Part model, mm, in its own coordinate system. Give positions to 0.01 mm unless a question says otherwise; leave off trailing zeros. Write each loop counter-clockwise with the first axis right and the second up, starting at its lowest first coordinate (ties: lowest second). Pieces come first, ordered by that corner, then holes.
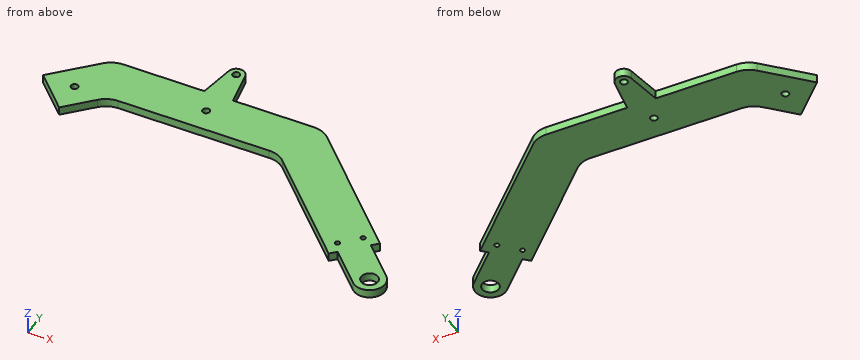
```python
from build123d import *

# Parameters (mm, degrees)
SKETCH5_R           = 1
SKETCH5_R_2         = 3.5
SKETCH5_R_3         = 1.5
BOSS_EXTRUDE1_DEPTH = 3.5
FILLET1_R           = 10


with BuildPart() as part:
    # Sketch5 → Boss-Extrude1 (new body)
    with BuildSketch(Plane.XY):
        with BuildLine():
            Line((91.161165235, 18.03122292), (104.596194078, 4.596194078))
            ThreePointArc((104.596194078, 4.596194078), (104.596194078, -4.596194078), (95.403805922, -4.596194078))
            Line((95.403805922, -4.596194078), (81.96877708, 8.838834765))
            Line((81.96877708, 8.838834765), (79.493903346, 6.363961031))
            Line((79.493903346, 6.363961031), (35.857864376, 50))
            Line((35.857864376, 50), (-35.857864376, 50))
            Line((-35.857864376, 50), (-49.445436483, 36.412427894))
            Line((-49.445436483, 36.412427894), (-63.587572106, 50.554563517))
            Line((-63.587572106, 50.554563517), (-44.142135624, 70))
            Line((-44.142135624, 70), (-6, 70))
            Line((-6, 70), (-3.448564481, 84.717831932))
            ThreePointArc((-3.448564481, 84.717831932), (0, 87.62), (3.448564481, 84.717831932))
            Line((3.448564481, 84.717831932), (6, 70))
            Line((6, 70), (44.142135624, 70))
            Line((44.142135624, 70), (93.636038969, 20.506096654))
            Line((93.636038969, 20.506096654), (91.161165235, 18.03122292))
        make_face()
        with Locations((86.564971157, 20.506096654)):
            Circle(SKETCH5_R, mode=Mode.SUBTRACT)
        with Locations((79.493903346, 13.435028843)):
            Circle(SKETCH5_R, mode=Mode.SUBTRACT)
        with Locations((100, 0)):
            Circle(SKETCH5_R_2, mode=Mode.SUBTRACT)
        with Locations((0, 84.12)):
            Circle(SKETCH5_R_3, mode=Mode.SUBTRACT)
        with Locations((0, 60)):
            Circle(SKETCH5_R_3, mode=Mode.SUBTRACT)
        with Locations((-50, 50)):
            Circle(SKETCH5_R_3, mode=Mode.SUBTRACT)
    extrude(amount=BOSS_EXTRUDE1_DEPTH)

    # Fillet1
    fillet1_edges = [part.edges().sort_by_distance(p)[0] for p in [
        (44.142135624, 70, 1.75),
        (35.857864376, 50, 1.75),
        (-35.857864376, 50, 1.75),
        (-44.142135624, 70, 1.75),
    ]]
    fillet(fillet1_edges, radius=FILLET1_R)


solid = part.part
```
1) Saw through at B-B, the plane z = 1.5. Write the cut outline in (x, y), then the cut area to 3 significant figures.
Answers follow:
outline: (-63.59, 50.55) - (-49.45, 36.41) - (-38.79, 47.07) arc R10 cw to (-31.72, 50) - (31.72, 50) arc R10 cw to (38.79, 47.07) - (79.49, 6.36) - (81.97, 8.84) - (95.4, -4.6) arc R6.5 ccw to (104.6, 4.6) - (91.16, 18.03) - (93.64, 20.51) - (47.07, 67.07) arc R10 ccw to (40, 70) - (6, 70) - (3.45, 84.72) arc R3.5 ccw to (-3.45, 84.72) - (-6, 70) - (-40, 70) arc R10 ccw to (-47.07, 67.07) - close; hole circle Ø3 at (-50, 50); hole circle Ø3 at (0, 60); hole circle Ø3 at (0, 84.12); hole circle Ø2 at (79.49, 13.44); hole circle Ø2 at (86.56, 20.51); hole circle Ø7 at (100, 0)
area: 3,790 mm2
2) Saw through at D-D, the plane y = 0. Write the cut outline in (x, z), then the cut area to 3 significant figures.
Answers follow:
outline: (90.81, 0) - (96.5, 0) - (96.5, 3.5) - (90.81, 3.5) - close; (103.5, 0) - (106.5, 0) - (106.5, 3.5) - (103.5, 3.5) - close
area: 30.4 mm2
3) Saw through at A-A, the plane y = 43.5. Write the cut outline in (x, z).
Answers follow:
outline: (-56.53, 0) - (-42.36, 0) - (-42.36, 3.5) - (-56.53, 3.5) - close; (42.36, 0) - (70.64, 0) - (70.64, 3.5) - (42.36, 3.5) - close
4) Pin check, flat tips, straight feed: pin 1 Ø2.5 at (x, y) = (86.56, 20.51) entering from -Z; pin 2 Ø1 at (x, z) = (-44, 3) entering from -Y; pin 3 Ø3 at (x, y) = (86, 31.5) entering from +Z; pin 4 Ø1.8 at (x, z) = (-27, 1.5) entering from +Y. Stop position of each tip, or through.
Answers follow:
pin 1: stops at z = 0
pin 2: stops at y = 41.36
pin 3: passes through
pin 4: stops at y = 70
5) Saw through at C-C, the plane x = 15. Write the cut outline in (y, z), then the cut area to 3 significant figures.
Answers follow:
outline: (50, 0) - (70, 0) - (70, 3.5) - (50, 3.5) - close
area: 70.0 mm2
6) Wall check: L1, parallel to Y at x = -25, z = 2.65; L2, parallel to Y at x = 100, z = 2.65; L3, parallel to X at y = -1.5, z = 2.8. Give the ranges that are in metal, low to high.
Answers follow:
L1: y = 50 to 70
L2: y = -6.5 to -3.5, 3.5 to 9.19
L3: x = 92.31 to 96.84, 103.16 to 106.32
